Autodesk Inventor part; units mm, degrees
ref_plane "YZ Plane" through (0, 0, 0) normal (1, 0, 0) x (0, 1, 0)
ref_plane "XZ Plane" through (0, 0, 0) normal (0, 1, 0) x (-1, 0, 0)
ref_plane "XY Plane" through (0, 0, 0) normal (0, 0, 1) x (1, 0, 0)
sketch "Sketch1" plane through (0, 0, 0) normal (0, 1, 0) x (-1, 0, 0)
  line L0 (-14.478, 12.7) -> (14.478, 12.7)
  line L1 (14.478, 12.7) -> (14.478, -12.7)
  line L2 (14.478, -12.7) -> (-14.478, -12.7)
  line L3 (-14.478, -12.7) -> (-14.478, 12.7)
  line L4 (-14.478, 12.7) -> (14.478, -12.7) construction
  line L5 (14.478, 12.7) -> (-14.478, -12.7) construction
  point P0 (0, 0)
  dimension "d0" = 28.956
  dimension "d1" = 25.4
extrude "Extrusion1" add sketch "Sketch1" along normal blind 12.7
sketch "Sketch2" plane through (0, 12.7, 0) normal (0, 1, 0) x (1, 0, 0)
  point P0 (0, 0)
  point P1 (0, -9.779)
  point P2 (0, 9.779)
  dimension "d4" = 9.779
  dimension "d5" = 19.558
hole "Hole1" at (0, 12.7, 9.779) at (0, 12.7, -9.779) direction (0, -1, 0) diameter 3.81 end through all
sketch "Sketch3" plane through (14.478, 0, 12.7) normal (1, 0, 0) x (0, 0, -1)
  circle A0 centre (12.7, 6.35) radius 1.5
  line L0 (25.4, 0) -> (0, 0)
  line L1 (0, 12.7) -> (25.4, 12.7)
  line L2 (11.582, 7.35) -> (13.818, 7.35)
  point P0 (12.7, 0)
  point P1 (12.7, 0)
  dimension "d13" = 3
  dimension "d14" = 6.35
  dimension "d15" = 12.7
  dimension "d18" = 1
extrude "Extrusion3" add sketch "Sketch3" along normal blind 9.7 contours A0 L2 picked at (12.7594, 6.5202)
sketch "Sketch4" plane through (0, 12.7, 0) normal (0, 1, 0) x (1, 0, 0)
  line L0 (-14.478, -2.1797) -> (-12.0814, -2.1797)
  line L1 (-12.0814, -2.1797) -> (-12.0814, 2.1797)
  line L2 (-12.0814, 2.1797) -> (-14.478, 2.1797)
  line L3 (-14.478, 2.1797) -> (-14.478, -2.1797)
  line L4 (-14.478, -2.1797) -> (-12.0814, 2.1797) construction
  line L5 (-12.0814, -2.1797) -> (-14.478, 2.1797) construction
  line L6 (-14.478, 12.7) -> (-14.478, -12.7)
  point P0 (0, 0)
  point P1 (-13.2797, 0)
  point P2 (-13.2797, 0)
extrude "Extrusion4" add sketch "Sketch4" along normal blind 6.35
properties part number "MotorWithEnclosure" material "ABS Plastic"
Check sheet for the modelled part. Datum: model origin and axes. Units: mm. A direction names the side the tool comes from. Give positions to 0.01 mm unless a question says otherwise; leave off trailing zeros. Loops run counter-clockwise (first coordinate to the right, second up) from the corner with the lowest first, then second, coordinate; pieces in that order, holes last. Notation, with made-up numbers: M 86,28.5 L 140,28.5 A18 cw 140,49.5 Z; hole C 67.5,-18 d10. An arc over 180 degrees is marked long. Answer as a JSON object with one key per item and string values. Group by question number.
Q1. Go/stop test with flat-tipped pins: P1, Ø6, axis at x = 0, z = -9.779, coming from the +Y side; P2, Ø8, axis at x = 0, z = 1.5, coming from the -Y side; P3, Ø0.7, axis at x = -13.5, y = 14.5, coming from the +Z side; P4, Ø3.5, axis at y = 15.5, z = -1, coming from the +X side. Record where each tip stops, or that it passes through.
Q2. Release check for a two-part mould opening along X. For faces 1 (the cylindrical face through (0.73, 6.26, -8.02)), 2 (the cylindrical face through (0.73, 6.26, 11.54)), 3 (the flat face through (-13, 16, 2.18)), 4 (the flat face through (14.478, 8, 0)) record: released by +X, released by -X, zero draft, split by the parting line, or undercut.
Q3. Cross-section at B-B on y = 6.35. Record the cut outline in (x, z) (3 decimals), then the cut area to 3 significant figures.
Q4. Cross-section at C-C on z = 0. Record the cut outline in (x, y).
Q5. Cross-section at D-D on z = -10.25. Record the cut outline in (x, y).
Q6. Material ranges on line 1 along Z through (x, y) = (0, 9); line 2 along Y through (x, z) = (14, 9.5); line 3 along X through (y, z) = (17.5, 1), recorded low to high. Write a range as [from, to].
Q7. Cross-section at A-A on x = 0. Record the cut outline in (y, z), then the cut area to 3 significant figures.
Q8. Access from +Z, -Z, +X, -X, +Y, -Y to the whole of each face (thin tool, end or side, straight path). Record for faces 5 (the flat face through (0, 6, -12.7)), 6 (the cylindrical face through (19.26, 4.85, -0.05)), 7 (the flat face through (-13, 16, -2.18)), 8 (the flat face through (19, 7.35, 0)).
Evaluation:
{
 "1": {"P1": "stops at y = 12.7", "P2": "stops at y = 0", "P3": "stops at z = 2.18", "P4": "stops at x = -12.08"},
 "2": {"face 1": "undercut", "face 2": "undercut", "face 3": "zero draft", "face 4": "released by +X"},
 "3": {"outline": "M -14.478,-12.7 L 14.478,-12.7 L 14.478,-1.5 L 24.178,-1.5 L 24.178,1.5 L 14.478,1.5 L 14.478,12.7 L -14.478,12.7 Z; hole C 0,-9.779 d3.81; hole C 0,9.779 d3.81", "area": "742 mm2"},
 "4": {"outline": "M -14.48,0 L 14.48,0 L 14.48,4.85 L 24.18,4.85 L 24.18,7.35 L 14.48,7.35 L 14.48,12.7 L -12.08,12.7 L -12.08,19.05 L -14.48,19.05 Z"},
 "5": {"outline": "M -14.48,0 L -1.85,0 L -1.85,12.7 L -14.48,12.7 Z; M 1.85,0 L 14.48,0 L 14.48,12.7 L 1.85,12.7 Z"},
 "6": {"line 1": "z = [-12.7, -11.68], [-7.87, 7.87], [11.68, 12.7]", "line 2": "y = [0, 12.7]", "line 3": "x = [-14.48, -12.08]"},
 "7": {"outline": "M 0,-12.7 L 12.7,-12.7 L 12.7,-11.68 L 0,-11.68 Z; M 0,-7.87 L 12.7,-7.87 L 12.7,7.87 L 0,7.87 Z; M 0,11.68 L 12.7,11.68 L 12.7,12.7 L 0,12.7 Z", "area": "226 mm2"},
 "8": {"face 5": "-Z, +X, -X, +Y, -Y", "face 6": "+X", "face 7": "-Z, +X, -X, +Y", "face 8": "+Z, -Z, +X, +Y"}
}
